Check sheet for the modelled part. Datum: model origin and axes. Units: mm. Round coordinates to 2 decimals unless told otherwise and drop trailing zeros. Write each loop counter-clockwise with the first axis right and the second up, starting at its lowest first coordinate (ties: lowest second). Pieces come first, ordered by that corner, then holes.
Item 1: Depth check by flat-ended pin: pin 1 (6 mm diameter, centred on y = -9.25, z = -273.685, fed in from -X); pin 2 (4 mm diameter, centred on y = -1, z = -80, fed in from +X) (3 decimals); pin 3 (1 mm diameter, centred on x = -46.5, y = -1.5, fed in from +Z). Enter the tip coordinate at first touch or a pass-through.
Item 2: Section check A-A, the plane z = 25. Record the cut outline in (x, y) (3 decimals).
Item 3: Material ranges on line 1 along Y through (x, z) = (-44.75, 192); line 2 along Y through (x, z) = (-44.75, 40.5); line 3 along Y through (x, z) = (-44.1, 99.59), recorded low to high.
from build123d import *

# Parameters (mm, degrees)
BOSS_EXTRUDE1_DEPTH                             = 281.94
BOSS_EXTRUDE1_DEPTH_BACK                        = 276.86
CBORE_FOR_M4_SHCS1_D                            = 4.5
CBORE_FOR_M4_SHCS1_CBORE_D                      = 8
CBORE_FOR_M4_SHCS1_CBORE_DEPTH                  = 4
CSK_FOR_M4_FLAT_HEAD_MACHINE_SCREW1_D           = 4.5
CSK_FOR_M4_FLAT_HEAD_MACHINE_SCREW1_CSINK_D     = 9.4
CSK_FOR_M4_FLAT_HEAD_MACHINE_SCREW1_CSINK_ANGLE = 90
LPATTERN1_COUNT                                 = 9
LPATTERN1_PITCH                                 = 60
LPATTERN1_COL_COUNT                             = 2
LPATTERN1_COL_PITCH                             = 60
CSK_FOR_6_FLAT_HEAD_MACHINE_SCREW1_D            = 3.7973
CSK_FOR_6_FLAT_HEAD_MACHINE_SCREW1_CSINK_D      = 7.0866
CSK_FOR_6_FLAT_HEAD_MACHINE_SCREW1_CSINK_ANGLE  = 82
CUT_EXTRUDE1_START                              = -5.775
CUT_EXTRUDE1_DEPTH                              = 5.775


with BuildPart() as part:
    # Sketch1 → Boss-Extrude1 (new, two sides: drawn at the far end of the back side and taken through both)
    with BuildSketch(Plane.XY.offset(-BOSS_EXTRUDE1_DEPTH_BACK)):
        Polygon((-39.1, 20), (-39.1, 11.75), (-40.375, 11.75), (-40.375, 18), (-44.875, 18), (-44.875, 6.25), (-41.875, 6.25), (-41.875, 5.5), (-43.125, 4.778312164), (-43.125, -4.778312164), (-41.875, -5.5), (-41.875, -6.25), (-44.875, -6.25), (-44.875, -18), (-40.375, -18), (-40.375, -11.75), (-39.1, -11.75), (-39.1, -20), (-47.625, -20), (-47.625, 20), align=None)
    extrude(amount=BOSS_EXTRUDE1_DEPTH + BOSS_EXTRUDE1_DEPTH_BACK)

    # CBORE for M4 SHCS1 (through all)
    with Locations(Plane(origin=(-43.125, 0, 0), x_dir=(0, 0, -1), z_dir=(1, 0, 0))):
        with Locations((-219.589999986, 0)):
            cbore_for_m4_shcs1 = CounterBoreHole(CBORE_FOR_M4_SHCS1_D / 2, CBORE_FOR_M4_SHCS1_CBORE_D / 2, CBORE_FOR_M4_SHCS1_CBORE_DEPTH)

    # CSK for M4 Flat Head Machine Screw1 (through all)
    with Locations(Plane(origin=(-47.625, 6.680483291, -0.93803287), x_dir=(0, 0, -1), z_dir=(-1, 0, 0))):
        with Locations((-241.52803302, 6.680483291), (-261.528032898, 6.680483291)):
            CounterSinkHole(CSK_FOR_M4_FLAT_HEAD_MACHINE_SCREW1_D / 2, CSK_FOR_M4_FLAT_HEAD_MACHINE_SCREW1_CSINK_D / 2, counter_sink_angle=CSK_FOR_M4_FLAT_HEAD_MACHINE_SCREW1_CSINK_ANGLE)

    # LPattern1: CBORE for M4 SHCS1 ×9
    with Locations(*[(0, 0, -i * LPATTERN1_PITCH) for i in range(1, LPATTERN1_COUNT)]):
        add(cbore_for_m4_shcs1, mode=Mode.SUBTRACT)

    # LPattern1 col: CBORE for M4 SHCS1 ×2
    with Locations(*[(0, 0, i * LPATTERN1_COL_PITCH) for i in range(1, LPATTERN1_COL_COUNT)]):
        add(cbore_for_m4_shcs1, mode=Mode.SUBTRACT)

    # CSK for #6 Flat Head Machine Screw1 (through all)
    with Locations(Plane(origin=(-47.625, 11.960142778, 21.111442158), x_dir=(0, 0, -1), z_dir=(-1, 0, 0))):
        with Locations((294.796442158, 21.210142874), (294.796442158, 2.710142682)):
            CounterSinkHole(CSK_FOR_6_FLAT_HEAD_MACHINE_SCREW1_D / 2, CSK_FOR_6_FLAT_HEAD_MACHINE_SCREW1_CSINK_D / 2, counter_sink_angle=CSK_FOR_6_FLAT_HEAD_MACHINE_SCREW1_CSINK_ANGLE)

    # Sketch8 → Cut-Extrude1 (cut)
    with BuildSketch(Plane(origin=(-39.1, 0, 0), x_dir=(0, 0, -1), z_dir=(1, 0, 0)).offset(CUT_EXTRUDE1_START)):
        with BuildLine():
            Line((271.300569415, -11.75), (276.86, -11.75))
            Line((276.86, -11.75), (276.86, 18))
            Line((276.86, 18), (270.51, 18))
            ThreePointArc((270.51, 18), (272.75506403, 17.07006403), (273.685, 14.825))
            ThreePointArc((273.685, 14.825), (272.75506403, 12.57993597), (270.51, 11.65))
            Line((270.51, 11.65), (270.51, -11.65))
            ThreePointArc((270.51, -11.65), (270.908434436, -11.675099208), (271.300569415, -11.75))
        make_face()
        with BuildLine():
            Line((270.51, -18), (276.86, -18))
            Line((276.86, -18), (276.86, -11.75))
            Line((276.86, -11.75), (271.300569415, -11.75))
            ThreePointArc((271.300569415, -11.75), (273.019051902, -12.879419482), (273.685, -14.825))
            ThreePointArc((273.685, -14.825), (272.75506403, -17.07006403), (270.51, -18))
        make_face()
        with BuildLine():
            ThreePointArc((269.719430585, -11.75), (267.360099208, -15.223434436), (270.51, -18))
            Line((270.51, -18), (270.51, -11.75))
            Line((270.51, -11.75), (269.719430585, -11.75))
        make_face()
        with BuildLine():
            Line((270.51, -11.75), (270.51, -18))
            ThreePointArc((270.51, -18), (272.75506403, -17.07006403), (273.685, -14.825))
            ThreePointArc((273.685, -14.825), (273.019051902, -12.879419482), (271.300569415, -11.75))
            Line((271.300569415, -11.75), (270.51, -11.75))
        make_face()
        with BuildLine():
            Line((269.719430585, -11.75), (270.51, -11.75))
            Line((270.51, -11.75), (270.51, -11.65))
            ThreePointArc((270.51, -11.65), (270.111565564, -11.675099208), (269.719430585, -11.75))
        make_face()
        with BuildLine():
            Line((270.51, -11.65), (270.51, -11.75))
            Line((270.51, -11.75), (271.300569415, -11.75))
            ThreePointArc((271.300569415, -11.75), (270.908434436, -11.675099208), (270.51, -11.65))
        make_face()
        with BuildLine():
            ThreePointArc((273.685, 14.825), (272.75506403, 17.07006403), (270.51, 18))
            Line((270.51, 18), (270.51, 11.65))
            ThreePointArc((270.51, 11.65), (272.75506403, 12.57993597), (273.685, 14.825))
        make_face()
        with BuildLine():
            Line((270.51, 11.65), (270.51, 18))
            ThreePointArc((270.51, 18), (267.335, 14.825), (270.51, 11.65))
        make_face()
    extrude(amount=CUT_EXTRUDE1_DEPTH, mode=Mode.SUBTRACT)


solid = part.part
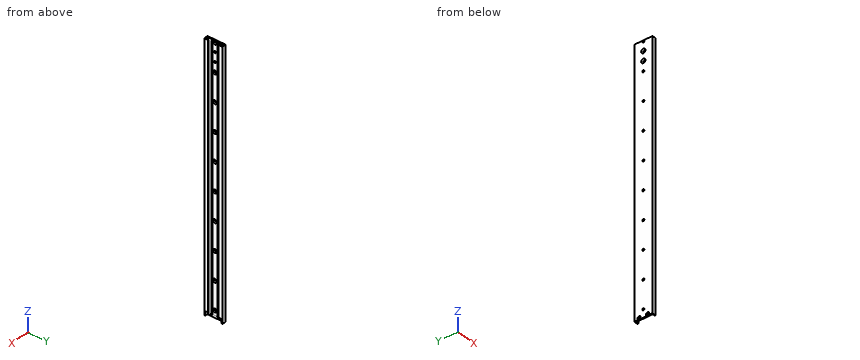
Values found:
1. pin 1: stops at x = -47
1. pin 2: stops at x = -47.125
1. pin 3: stops at z = 276.13
2. outline: (-47.625, -20) - (-39.1, -20) - (-39.1, -11.75) - (-40.375, -11.75) - (-40.375, -18) - (-44.875, -18) - (-44.875, -6.25) - (-41.875, -6.25) - (-41.875, -5.5) - (-43.125, -4.778) - (-43.125, 4.778) - (-41.875, 5.5) - (-41.875, 6.25) - (-44.875, 6.25) - (-44.875, 18) - (-40.375, 18) - (-40.375, 11.75) - (-39.1, 11.75) - (-39.1, 20) - (-47.625, 20) - close
3. line 1: y = -20 to -18, -6.25 to 6.25, 18 to 20
3. line 2: y = -20 to -18, -6.25 to -3.9, 3.9 to 6.25, 18 to 20
3. line 3: y = -20 to -18, -6.25 to -4, 4 to 6.25, 18 to 20
